Autodesk Inventor part; units mm, degrees
ref_plane "YZ Plane" through (0, 0, 0) normal (1, 0, 0) x (0, 1, 0)
ref_plane "XZ Plane" through (0, 0, 0) normal (0, 1, 0) x (-1, 0, 0)
ref_plane "XY Plane" through (0, 0, 0) normal (0, 0, 1) x (1, 0, 0)
sketch "Esquisse1" plane through (0, 0, 0) normal (0, 0, 1) x (1, 0, 0)
  line L0 (0, 0) -> (80, 0)
  line L1 (80, 0) -> (80, 550)
  line L2 (80, 550) -> (0, 550)
  line L3 (0, 550) -> (0, 0)
  dimension "d0" = 80
  dimension "d1" = 550
extrude "Extrusion1" add sketch "Esquisse1" along normal blind 21
chamfer "Chanfrein1" distance 5 angle 45 2 edges at (0, 550, 10.5) (80, 550, 10.5)
sketch "Esquisse4" plane through (0, 0, 21) normal (0, 0, 1) x (1, 0, 0)
  line L0 (0, 545) -> (0, 0)
  line L1 (80, 0) -> (80, 545)
  line L2 (0, 80) -> (29.1176, 0)
  line L3 (0, 0) -> (80, 0)
  line L4 (50.8824, 0) -> (80, 80)
  line L5 (29.1176, 0) -> (50.8824, 0)
  line L6 (30, 98.55) -> (50, 98.55)
  line L7 (50, 98.55) -> (50, 80)
  line L8 (50, 80) -> (30, 80)
  line L9 (30, 80) -> (30, 98.55)
  line L10 (40, 0) -> (40, 80) construction
  dimension "d23" = 70
  dimension "d24" = 70
  dimension "d25" = 80
  dimension "d26" = 20
  dimension "d27" = 18.55
extrude "Extrusion3" cut sketch "Esquisse4" against normal blind 21
sketch "Esquisse6" plane through (0, 0, 21) normal (0, 0, 1) x (1, 0, 0)
  line L0 (75, 550) -> (5, 550) construction
  line L1 (35, 520) -> (35, 545)
  line L2 (0, 545) -> (0, 80) construction
  line L3 (0, 535) -> (35, 535) construction
  line L4 (45, 535) -> (80, 535) construction
  line L5 (80, 80) -> (80, 545) construction
  line L6 (25, 270) -> (25, 520)
  line L7 (25, 520) -> (35, 520)
  line L8 (25, 395) -> (0, 395) construction
  line L9 (55, 395) -> (80, 395) construction
  line L10 (40, 550) -> (40, 270) construction
  line L11 (25, 270) -> (40, 270)
  line L12 (40, 270) -> (40, 550)
  line L13 (35, 545) -> (25, 545)
  line L14 (25, 545) -> (25, 550)
  line L15 (25, 550) -> (40, 550)
  point P0 (0, 0)
  point P1 (35, 550)
  dimension "d39" = 5
  dimension "d41" = 30
  dimension "d42" = 250
  dimension "d43" = 15
  dimension "d45" = 5
  dimension "d46" = 15
revolve "Révolution1" [suppressed]
properties part number "graduated_foot_03"
Here's how the part is built. I have some questions about the finished solid (model axes, mm). A direction names the side the tool comes from. Coordinates: 2 decimals unless noted, no trailing zeros. Order: outer loops, then holes, each group sorted by start corner. A loop starts at its lowest first (then second) coordinate and runs counter-clockwise, first axis right, second up. Notation, with made-up numbers: M 57,17 L 103,17 A11 ccw 103,25 Z; hole C 76,-35 d1. An arc over 180 degrees is marked long. Answer as a JSON object with one key per item and string values. Group by question number.
(1) I need wall thicknesses on probe 1 along X at (y, z) = (98, 12); probe 2 along Y at (x, z) = (49.5, 3.75). Which ranges of each line are inside material? Lowest first, please.
(2) For pin 1 (10 mm diameter, centred on x = 44, z = 12, fed in from -Y), with a flat end and sliding along its axis, tell me the tip position at first contact or that it passes through.
(3) Suppose I cut it at D-D, the plane x = 66. Please give me the cut outline in (y, z), then the cut area to 3 significant figures.
(4) Suppose I cut it at C-C, the plane y = 54.5. Please give me the cut outline in (x, z), then the cut area to 3 significant figures.
(5) Suppose I cut it at B-B, the plane z = 5.75. Please give me the cut outline in (x, y).
(6) Suppose I cut it at A-A, the plane x = 40.5. Please give me the cut outline in (y, z).
(7) Which directions (+Z, -Z, +X, -X, +Y, -Y) give clear straight access to the entire face, cutting with the end or side of a thin tool? Please do faces 1 (the face through (65.237, 39.44, 10.647)), 2 (the face through (40, 98.55, 11)).
(8) If we mould it in two halves opening along X, with no side actions, what happens to faces 3 (the face through (14.355, 40.56, 10.647)), 4 (the face through (80, 309, 10)), 5 (the face through (40, 80, 11)), 6 (the face through (39, 279, 21))? For each: released by +X, released by -X, zero draft, split by the parting line, or undercut.
Values found:
{
 "1": {"probe 1": "x = 0 to 30, 50 to 80", "probe 2": "y = 0 to 80, 98.55 to 550"},
 "2": {"pin 1": "stops at y = 0"},
 "3": {"outline": "M 41.54,0 L 550,0 L 550,21 L 41.54,21 Z", "area": "10,700 mm^2"},
 "4": {"outline": "M 9.28,0 L 70.72,0 L 70.72,21 L 9.28,21 Z", "area": "1,290 mm^2"},
 "5": {"outline": "M 0,80 L 29.12,0 L 50.88,0 L 80,80 L 80,545 L 75,550 L 5,550 L 0,545 Z; hole M 30,80 L 50,80 L 50,98.55 L 30,98.55 Z"},
 "6": {"outline": "M 0,0 L 80,0 L 80,21 L 0,21 Z; M 98.55,0 L 550,0 L 550,21 L 98.55,21 Z"},
 "7": {"face 1": "+Z, -Z, +X, -Y", "face 2": "+Z, -Z"},
 "8": {"face 3": "released by -X", "face 4": "released by +X", "face 5": "undercut", "face 6": "zero draft"}
}
